Verification items for the finished model (mm, model axes). Round coordinates to 2 decimals unless told otherwise and drop trailing zeros. Write each loop counter-clockwise with the first axis right and the second up, starting at its lowest first coordinate (ties: lowest second). Pieces come first, ordered by that corner, then holes. Notation, with made-up numbers: M 40.5,48 L 99.5,48 A24 cw 99.5,68 Z; hole C 3.25,-21 d5. An arc over 180 degrees is marked long. One line per item, written item: value. Start each with the question number.
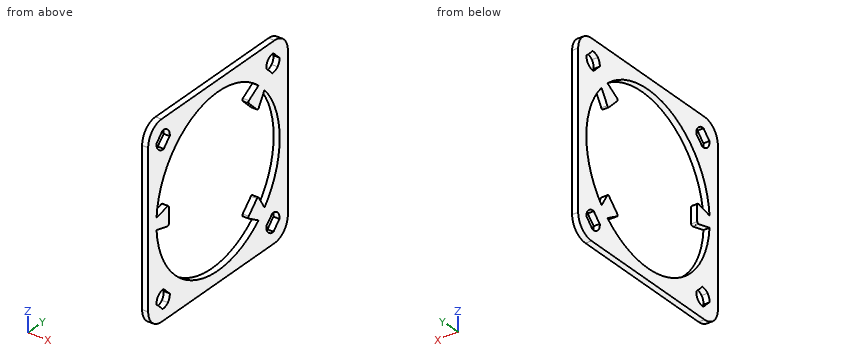
Autodesk Inventor part; units mm, degrees
ref_plane "YZ Plane" through (0, 0, 0) normal (1, 0, 0) x (0, 1, 0)
ref_plane "XZ Plane" through (0, 0, 0) normal (0, 1, 0) x (-1, 0, 0)
ref_plane "XY Plane" through (0, 0, 0) normal (0, 0, 1) x (1, 0, 0)
sketch "Sketch1" plane through (0, 0, 0) normal (1, 0, 0) x (0, 1, 0)
  line L0 (-12.75, 15.75) -> (12.75, 15.75)
  line L1 (15.75, 12.75) -> (15.75, -12.75)
  line L2 (12.75, -15.75) -> (-12.75, -15.75)
  line L3 (-15.75, -12.75) -> (-15.75, 12.75)
  line L4 (-15.75, 15.75) -> (15.75, -15.75) construction
  line L5 (15.75, 15.75) -> (-15.75, -15.75) construction
  line L6 (15.75, 15.75) -> (-15.75, -15.75)
  line L7 (7.9011, 23.5989) -> (-23.5989, -7.9011)
  circle A0 centre (0, 0) radius 17.5 construction
  line L8 (28.1244, 3.3756) -> (-3.3756, -28.1244) construction
  arc A1 (10.8821, -12.2221) -> (11.3137, -13.435) centre (12.3744, -12.3744) ccw
  arc A2 (13.435, -11.3137) -> (12.2221, -10.8821) centre (12.3744, -12.3744) ccw
  arc A3 (10.8821, -12.2221) -> (12.2221, -10.8821) centre (0, 0) ccw
  arc A4 (11.3137, -13.435) -> (12.5266, -13.8666) centre (12.3744, -12.3744) ccw
  arc A5 (13.8666, -12.5266) -> (13.435, -11.3137) centre (12.3744, -12.3744) ccw
  arc A6 (13.8666, -12.5266) -> (12.5266, -13.8666) centre (24.7487, -24.7487) ccw
  arc A7 (12.5266, 13.8666) -> (11.3137, 13.435) centre (12.3744, 12.3744) ccw
  arc A8 (12.5266, 13.8666) -> (13.8666, 12.5266) centre (24.7487, 24.7487) ccw
  arc A9 (13.435, 11.3137) -> (13.8666, 12.5266) centre (12.3744, 12.3744) ccw
  arc A10 (12.2221, 10.8821) -> (13.435, 11.3137) centre (12.3744, 12.3744) ccw
  arc A11 (12.2221, 10.8821) -> (10.8821, 12.2221) centre (0, 0) ccw
  arc A12 (11.3137, 13.435) -> (10.8821, 12.2221) centre (12.3744, 12.3744) ccw
  arc A13 (-13.8666, 12.5266) -> (-13.435, 11.3137) centre (-12.3744, 12.3744) ccw
  arc A14 (-13.8666, 12.5266) -> (-12.5266, 13.8666) centre (-24.7487, 24.7487) ccw
  arc A15 (-11.3137, 13.435) -> (-12.5266, 13.8666) centre (-12.3744, 12.3744) ccw
  arc A16 (-10.8821, 12.2221) -> (-11.3137, 13.435) centre (-12.3744, 12.3744) ccw
  arc A17 (-10.8821, 12.2221) -> (-12.2221, 10.8821) centre (0, 0) ccw
  arc A18 (-13.435, 11.3137) -> (-12.2221, 10.8821) centre (-12.3744, 12.3744) ccw
  arc A19 (-12.5266, -13.8666) -> (-11.3137, -13.435) centre (-12.3744, -12.3744) ccw
  arc A20 (-12.5266, -13.8666) -> (-13.8666, -12.5266) centre (-24.7487, -24.7487) ccw
  arc A21 (-13.435, -11.3137) -> (-13.8666, -12.5266) centre (-12.3744, -12.3744) ccw
  arc A22 (-12.2221, -10.8821) -> (-13.435, -11.3137) centre (-12.3744, -12.3744) ccw
  arc A23 (-12.2221, -10.8821) -> (-10.8821, -12.2221) centre (0, 0) ccw
  arc A24 (-11.3137, -13.435) -> (-10.8821, -12.2221) centre (-12.3744, -12.3744) ccw
  arc A25 (15.75, 12.75) -> (12.75, 15.75) centre (12.75, 12.75) ccw
  arc A26 (-12.75, 15.75) -> (-15.75, 12.75) centre (-12.75, 12.75) ccw
  arc A27 (-15.75, -12.75) -> (-12.75, -15.75) centre (-12.75, -12.75) ccw
  arc A28 (12.75, -15.75) -> (15.75, -12.75) centre (12.75, -12.75) ccw
  line L9 (9.1716, -6.9652) -> (10.4759, -9.1359)
  line L10 (-15.0803, 16.4203) -> (16.4197, -15.0797) construction
  line L11 (6.9652, -9.1716) -> (9.1359, -10.4759)
  line L12 (-16.4203, 15.0803) -> (15.0797, -16.4197) construction
  line L13 (23.5989, 7.9011) -> (15.75, 0.0522)
  line L14 (8.7806, -6.9172) -> (6.9172, -8.7806)
  arc A29 (9.1716, -6.9652) -> (8.7806, -6.9172) centre (8.9573, -7.094) ccw
  arc A30 (6.9172, -8.7806) -> (6.9652, -9.1716) centre (7.094, -8.9573) ccw
  line L15 (9.1716, 6.9652) -> (10.4759, 9.1359)
  arc A31 (8.7806, 6.9172) -> (9.1716, 6.9652) centre (8.9573, 7.094) ccw
  line L16 (6.9172, 8.7806) -> (8.7806, 6.9172)
  arc A32 (6.9652, 9.1716) -> (6.9172, 8.7806) centre (7.094, 8.9573) ccw
  line L17 (6.9652, 9.1716) -> (9.1359, 10.4759)
  line L18 (-11.4105, 1.5602) -> (-13.8677, 0.9475)
  arc A33 (-11.1, 1.3176) -> (-11.4105, 1.5602) centre (-11.35, 1.3176) ccw
  arc A34 (-11.4105, -1.5602) -> (-11.1, -1.3176) centre (-11.35, -1.3176) ccw
  line L19 (-11.1, -1.3176) -> (-11.1, 1.3176)
  line L20 (-11.4105, -1.5602) -> (-13.8677, -0.9475)
  arc A35 (10.4759, -9.1359) -> (10.4759, 9.1359) centre (0, 0) ccw
  arc A36 (9.1359, 10.4759) -> (-13.8677, 0.9475) centre (0, 0) ccw
  arc A37 (-13.8677, -0.9475) -> (9.1359, -10.4759) centre (0, 0) ccw
  point P0 (9.0068, -6.691)
  point P1 (6.691, -9.0068)
  point P2 (9.0068, 6.691)
  point P3 (6.691, 9.0068)
  point P4 (-11.1, 1.6376)
  point P5 (-11.1, -1.6376)
  dimension "d10" = 35
  dimension "d0" = 31.5
  dimension "d1" = 31.5
  dimension "d4" = 11.1
  dimension "d17" = 360
  dimension "d19" = 3
  dimension "d21" = 0.25
  dimension "d22" = 0.25
  dimension "d25" = 90
  dimension "d29" = 135
extrude "Extrusion1" add sketch "Sketch1" along normal blind 1 contours L0 L7 A36 L3 A26 | L0 A25 L6 A8 A7 A12 A11 L16 A32 L17 A36 L7 | L7 A36 L18 A33 L19 A34 L20 A37 L6 A23 A22 A21 A20 A27 L3 | A25 L1 A28 L2 A27 L6 A20 A19 A24 A23 A37 L11 A30 L14 A29 L9 A35 L15 A31 L16 A11 A10 A9 A8
properties part number "Harting Gasket 1"
1) Cross-section at A-A (y = -9). Record the boundary of the cut face in (x, z), then the cut area to 3 significant figures.
2) Thickness scan on line 1 (Z direction, x = 0.9, y = -11.5); line 2 (Y direction, x = 0.5, z = 11). Record the ranges inside material, lowest first.
3) Cross-section at D-D (z = 8). Record the boundary of the cut face in (x, y), then the cut area to 3 significant figures.
4) Cross-section at B-B (z = 3). Record the boundary of the cut face in (x, y).
5) Cross-section at C-C (x = 0.8). State how many separate pieces and enclosed holes the cut face has, then the cut area to 3 significant figures.
Results below:
1. outline: M 0,-15.75 L 1,-15.75 L 1,-10.59 L 0,-10.59 Z; M 0,10.59 L 1,10.59 L 1,15.75 L 0,15.75 Z
1. area: 10.3 mm²
2. line 1: z = -15.75 to -13.59, -11.64 to -7.81, -1.54 to 1.54, 7.81 to 11.64, 13.59 to 15.75
2. line 2: y = -15.75 to -12.98, -12.12 to -8.5, 8.5 to 12.12, 12.98 to 15.75
3. outline: M 0,-15.75 L 1,-15.75 L 1,-11.37 L 0,-11.37 Z; M 0,7.7 L 1,7.7 L 1,9.79 L 0,9.79 Z; M 0,11.37 L 1,11.37 L 1,15.75 L 0,15.75 Z
3. area: 10.9 mm²
4. outline: M 0,-15.75 L 1,-15.75 L 1,-13.57 L 0,-13.57 Z; M 0,13.57 L 1,13.57 L 1,15.75 L 0,15.75 Z
5. separate pieces: 1
5. enclosed holes: 5
5. area: 374 mm²
